Read the model definition and answer for the solid it produces. Units are mm, in the model's axes. A direction names the side the tool comes from. Give positions to 0.01 mm unless a question says otherwise; leave off trailing zeros. Write each loop counter-clockwise with the first axis right and the second up, starting at its lowest first coordinate (ties: lowest second). Pieces come first, ordered by that corner, then holes. Notation, with made-up numbers: (27, -40) -> (71, -40) arc R22 ccw to (71, -3) -> close; hole circle Ø9 at (57.25, -27). An arc over 180 degrees is marked (long way). Answer as CSV lines item,"result". Start each with the question number.
1. For a pull along X with two mould halves and no side action, classify faces 3 (the cylindrical face through (54, 39, 1)), 4 (the flat face through (55, 28, 0)) as pulls with the +X half, pulls with the -X half, needs draft (parallel to the pull), parting line crosses it, or undercut.
2. The part is cut by section C-C, the plane z = 1.15. Give the number of separate pieces and of enclosed holes in the cut face, and give its area (3 significant figures).
3. The part is cut by section A-A, the plane x = 44. Determine the outline of the cut face in (y, z), and give its area (3 significant figures).
4. The part is cut by section D-D, the plane x = 85.5. Determine the outline of the cut face in (y, z).
5. A tool of negligible diameter and unlimited length cuts with its end or side. For faces 1 (the flat face through (59, -2, 1)), 2 (the cylindrical face through (39, 39, 1)), from which of +Z, -Z, +X, -X, +Y, -Y can it reach the whole face along a straight path? Write none if from no direction.
6. Given pin 1 (1 mm diameter, centred on x = 45.5, z = 0.5, fed in from -Y); pin 2 (0.6 mm diameter, centred on x = 67.5, z = 1.5, fed in from +Y); pin 3 (0.6 mm diameter, centred on y = 43, z = 0.5, fed in from +X), each flat-ended and moving along its own axis, determine where each tip first touches the part or whether it passes through.
7. Find the intervals of material crossed by line 1 (Y direction, x = 74.5, z = 1.95); line 2 (X direction, y = 53, z = 0.95), in increasing order.
8. The part is cut by section B-B, the plane y = 23. Determine the outline of the cut face in (x, z).
from build123d import *

# Parameters (mm, degrees)
SKETCH_1_W             = 95
SKETCH_1_H             = 56
EXTRUDE_1_DEPTH        = 2
SKETCH_3_W             = 13.5
SKETCH_3_H             = 56
CUT_EXTRUDE_2_DEPTH    = 111.29505882
CUT_EXTRUDE_4_DEPTH    = 111.29505882
PATTERN_LINEAR_1_COUNT = 10
PATTERN_LINEAR_1_PITCH = 5
SKETCH_10_W            = 7
SKETCH_10_H            = 2
EXTRUDE_2_DEPTH        = 2
SKETCH_11_R            = 0.5
CUT_EXTRUDE_7_DEPTH    = 112.323851892
SKETCH_13_W            = 2
SKETCH_13_H            = 7
EXTRUDE_4_DEPTH        = 2
SKETCH_14_R            = 0.5
CUT_EXTRUDE_8_DEPTH    = 114.035392687


with BuildPart() as part:
    # 草图1 → 凸台-拉伸1 (new body)
    with BuildSketch(Plane.XY):
        with Locations((47.5, 28)):
            Rectangle(SKETCH_1_W, SKETCH_1_H)
    extrude(amount=EXTRUDE_1_DEPTH)

    # 草图3 → 切除-拉伸2 (cut, through all)
    with BuildSketch(Plane(origin=(0, 0, 0), x_dir=(-1, 0, 0), z_dir=(0, 0, -1))):
        with Locations((-6.75, 28)):
            Rectangle(SKETCH_3_W, SKETCH_3_H)
    extrude(amount=-CUT_EXTRUDE_2_DEPTH, mode=Mode.SUBTRACT)

    # 草图6 → 切除-拉伸4 (cut, through all)
    with BuildSketch(Plane(origin=(0, 0, 0), x_dir=(-1, 0, 0), z_dir=(0, 0, -1))):
        with BuildLine():
            Line((-63, 50), (-63, 40))
            ThreePointArc((-63, 40), (-64, 39), (-65, 40))
            Line((-65, 40), (-65, 50))
            ThreePointArc((-65, 50), (-64, 51), (-63, 50))
        make_face()
    cut_extrude_4 = extrude(amount=-CUT_EXTRUDE_4_DEPTH, mode=Mode.SUBTRACT)

    # 阵列(线性)1: 切除-拉伸4 ×10
    with Locations(*[(-i * PATTERN_LINEAR_1_PITCH, 0, 0) for i in range(1, PATTERN_LINEAR_1_COUNT)]):
        add(cut_extrude_4, mode=Mode.SUBTRACT)

    # 草图10 → 凸台-拉伸2 (add)
    with BuildSketch(Plane(origin=(0, 0, 0), x_dir=(-1, 0, 0), z_dir=(0, 0, -1))):
        with Locations((-36.5, 57)):
            Rectangle(SKETCH_10_W, SKETCH_10_H)
        with Locations((-80.5, 57)):
            Rectangle(SKETCH_10_W, SKETCH_10_H)
        with Locations((-58.5, 57)):
            Rectangle(SKETCH_10_W, SKETCH_10_H)
        with Locations((-80.5, -1)):
            Rectangle(SKETCH_10_W, SKETCH_10_H)
        with Locations((-58.5, -1)):
            Rectangle(SKETCH_10_W, SKETCH_10_H)
        with Locations((-36.5, -1)):
            Rectangle(SKETCH_10_W, SKETCH_10_H)
    extrude(amount=-EXTRUDE_2_DEPTH)

    # 草图11 → 切除-拉伸7 (cut, through all)
    with BuildSketch(Plane(origin=(0, 0, 0), x_dir=(-1, 0, 0), z_dir=(0, 0, -1))):
        with Locations((-84, 56)):
            Circle(SKETCH_11_R)
        with Locations((-77, 56)):
            Circle(SKETCH_11_R)
        with Locations((-62, 56)):
            Circle(SKETCH_11_R)
        with Locations((-55, 56)):
            Circle(SKETCH_11_R)
        with Locations((-40, 56)):
            Circle(SKETCH_11_R)
        with Locations((-33, 56)):
            Circle(SKETCH_11_R)
        with Locations((-84, 0)):
            Circle(SKETCH_11_R)
        with Locations((-77, 0)):
            Circle(SKETCH_11_R)
        with Locations((-62, 0)):
            Circle(SKETCH_11_R)
        with Locations((-55, 0)):
            Circle(SKETCH_11_R)
        with Locations((-40, 0)):
            Circle(SKETCH_11_R)
        with Locations((-33, 0)):
            Circle(SKETCH_11_R)
    extrude(amount=-CUT_EXTRUDE_7_DEPTH, mode=Mode.SUBTRACT)

    # 草图13 → 凸台-拉伸4 (add)
    with BuildSketch(Plane(origin=(0, 0, 0), x_dir=(-1, 0, 0), z_dir=(0, 0, -1))):
        with Locations((-96, 13.5)):
            Rectangle(SKETCH_13_W, SKETCH_13_H)
        with Locations((-96, 35.5)):
            Rectangle(SKETCH_13_W, SKETCH_13_H)
    extrude(amount=-EXTRUDE_4_DEPTH)

    # 草图14 → 切除-拉伸8 (cut, through all)
    with BuildSketch(Plane(origin=(0, 0, 0), x_dir=(-1, 0, 0), z_dir=(0, 0, -1))):
        with Locations((-95, 39)):
            Circle(SKETCH_14_R)
        with Locations((-95, 32)):
            Circle(SKETCH_14_R)
        with Locations((-95, 17)):
            Circle(SKETCH_14_R)
        with Locations((-95, 10)):
            Circle(SKETCH_14_R)
    extrude(amount=-CUT_EXTRUDE_8_DEPTH, mode=Mode.SUBTRACT)


solid = part.part
Results found:
1,face 3,"undercut"
1,face 4,"needs draft"
2,separate pieces,"1"
2,enclosed holes,"10"
2,area,"4,440 mm²"
3,outline,"(0, 0) -> (39, 0) -> (39, 2) -> (0, 2) -> close; (51, 0) -> (56, 0) -> (56, 2) -> (51, 2) -> close"
3,area,"88.0 mm²"
4,outline,"(0, 0) -> (56, 0) -> (56, 2) -> (0, 2) -> close"
5,face 1,"+Z, -Z, +X, -X, -Y"
5,face 2,"+Z, -Z"
6,pin 1,"stops at y = 0"
6,pin 2,"stops at y = 56"
6,pin 3,"stops at x = 95"
7,line 1,"y = 0 to 56"
7,line 2,"x = 13.5 to 95"
8,outline,"(13.5, 0) -> (95, 0) -> (95, 2) -> (13.5, 2) -> close"
